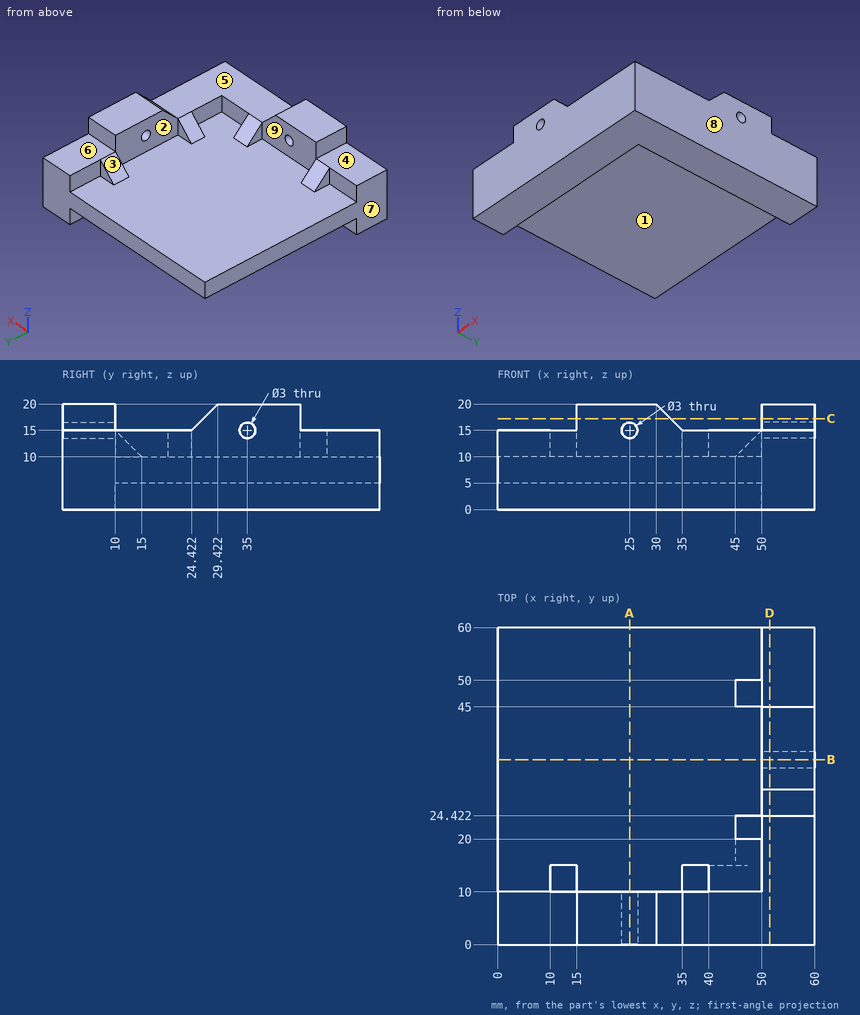
Study the drawing (mm; zero at the part's minimum x, y, z) and answer. A direction names the side the tool comes from. Coordinates: 2 decimals unless noted, no trailing zeros. Write each loop counter-clockwise with the first axis right and the second up, starting at its lowest first coordinate (ties: lowest second). Pieces come first, ordered by that corner, then holes. Notation, with made-up numbers: (8, 60) - (64, 60) arc R23 ccw to (64, 89) - close; hole circle Ø9 at (37.25, 60). An arc over 180 degrees is marked (long way). Return JSON: item names as keys, results as strings. Group by question number.
1. A cutting plane is placed at D-D, the plane x = 51.5. Determine the outline of the cut face in (y, z).
2. Determine the mould class of the marked faces 6, 7, 8 and 9 for opening direction X: released by +X, released by -X, zero draft, split by the parting line, or undercut.
3. A cutting plane is placed at B-B, the plane y = 35. Determine the outline of the cut face in (x, z), plus the area to 3 significant figures.
4. Given pin 1 (8 mm diameter, centred on y = 32, z = 13.5, fed in from -X); pin 2 (3.5 mm diameter, centred on y = 35, z = 15, fed in from -X); pin 3 (1 mm diameter, centred on x = 40, y = 23.5, fed in from -Z); pin 4 (4 mm diameter, centred on x = 25.5, y = 43.5, fed in from +Z), each flat-ended and moving along its own axis, determine where each tip first touches the part or whether it passes through.
5. Which of the six approach directions +Z, -Z, +X, -X, +Y, -Y give full straight-line access (tool end or side, diameter ignored) to the marked faces 1, 2, 3, 4 and 5?
6. A cutting plane is placed at A-A, the plane x = 25. Determine the outline of the cut face in (y, z), plus the area to 3 significant figures.
7. Straight lines are drawn through the part: L1, parallel to X at y = 13, z = 11.25; L2, parallel to Z at x = 25, y = 6.5; L3, parallel to Z at x = 21, y = 32. For each, find the intervals that lie inside material, in ascending order.
8. A cutting plane is placed at C-C, the plane z = 17.25. Determine the outline of the cut face in (x, y).
Ans:
{
 "1": {"outline": "(0, 0) - (60, 0) - (60, 15) - (45, 15) - (45, 20) - (29.42, 20) - (24.42, 15) - (0, 15) - close; hole circle Ø3 at (35, 15)"},
 "2": {"face 6": "zero draft", "face 7": "released by -X", "face 8": "released by +X", "face 9": "undercut"},
 "3": {"outline": "(0, 5) - (50, 5) - (50, 0) - (60, 0) - (60, 13.5) - (50, 13.5) - (50, 10) - (0, 10) - close; (50, 16.5) - (60, 16.5) - (60, 20) - (50, 20) - close", "area": "420 mm²"},
 "4": {"pin 1": "x = 0", "pin 2": "x = 50", "pin 3": "z = 5", "pin 4": "z = 10"},
 "5": {"face 1": "-Z, -X, +Y", "face 2": "+Z, -X", "face 3": "+Z, -X, +Y", "face 4": "+Z, -X, +Y, -Y", "face 5": "+Z, +X, -Y"},
 "6": {"outline": "(0, 0) - (10, 0) - (10, 5) - (60, 5) - (60, 10) - (10, 10) - (10, 13.5) - (0, 13.5) - close; (0, 16.5) - (10, 16.5) - (10, 20) - (0, 20) - close", "area": "420 mm²"},
 "7": {"L1": "10 to 15, 35 to 40, 50 to 60", "L2": "0 to 13.5, 16.5 to 20", "L3": "5 to 10"},
 "8": {"outline": "(15, 0) - (32.75, 0) - (32.75, 10) - (15, 10) - close; (50, 26.67) - (60, 26.67) - (60, 45) - (50, 45) - close"}
}
